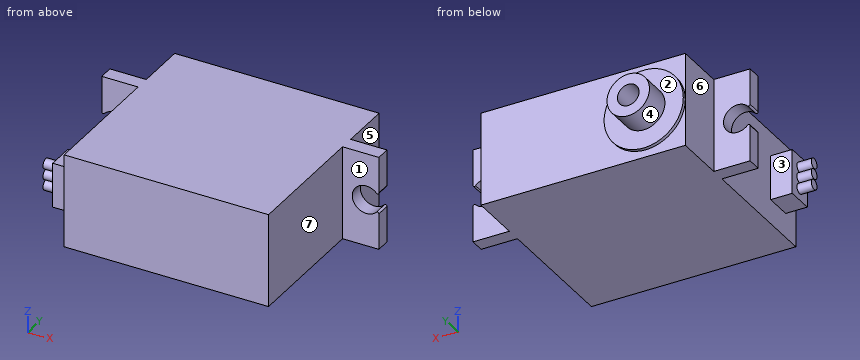
from build123d import *

# Parameters (mm, degrees)
ESQUISSE1_W                       = 28.4
ESQUISSE1_H                       = 27.2
ESQUISSE1_W_2                     = 5.05
ESQUISSE1_H_2                     = 2
BOSS_EXTRU_1_DEPTH                = 6.5
DIAM_TRE_DU_PER_AGE_3_9_3_9_1_D   = 3.9
CONG_1_R                          = 0.2
ESQUISSE6_R                       = 5.5
BOSS_EXTRU_4_DEPTH                = 0.5
ESQUISSE4_R                       = 2.95
BOSS_EXTRU_2_DEPTH                = 3.8
DIAM_TRE_DU_PER_AGE_3_0_3_1_D     = 3
DIAM_TRE_DU_PER_AGE_3_0_3_1_DEPTH = 6
DIAM_TRE_DU_PER_AGE_3_0_3_1_TIP   = 0.901290929
ESQUISSE8_W                       = 6.2
ESQUISSE8_H                       = 3.7
BOSS_EXTRU_5_DEPTH                = 3
ESQUISSE9_R                       = 0.7
BOSS_EXTRU_6_DEPTH                = 2


with BuildPart() as part:
    # Esquisse1 → Boss.-Extru.1 (new, symmetric)
    with BuildSketch(Plane.XY):
        with Locations((0, -4.6)):
            Rectangle(ESQUISSE1_W, ESQUISSE1_H)
        with Locations((-16.725, 1)):
            Rectangle(ESQUISSE1_W_2, ESQUISSE1_H_2)
        with Locations((16.725, 1)):
            Rectangle(ESQUISSE1_W_2, ESQUISSE1_H_2)
    extrude(amount=BOSS_EXTRU_1_DEPTH, both=True)

    # Diamètre du perçage Ø3.9 (3.9)1 (through all)
    with Locations(Plane(origin=(0, 2, 0), x_dir=(1, 0, 0), z_dir=(0, 1, 0))):
        with Locations((-17.5, 0), (17.5, 0)):
            Hole(DIAM_TRE_DU_PER_AGE_3_9_3_9_1_D / 2)

    # Congé1
    cong_1_edges = [part.edges().sort_by_distance(p)[0] for p in [
        (19.25, 1, -0.860232527),
        (19.25, 1, 0.860232527),
        (-19.25, 1, -0.860232527),
        (-19.25, 1, 0.860232527),
    ]]
    fillet(cong_1_edges, radius=CONG_1_R)

    # Esquisse6 → Boss.-Extru.4 (add)
    with BuildSketch(Plane(origin=(0, 9, 0), x_dir=(1, 0, 0), z_dir=(0, 1, 0))):
        with Locations(Location((-8.7, 0, 0), (0, 0, 180))):
            Circle(ESQUISSE6_R)
    extrude(amount=BOSS_EXTRU_4_DEPTH)

    # Esquisse4 → Boss.-Extru.2 (add)
    with BuildSketch(Plane(origin=(0, 9.5, 0), x_dir=(1, 0, 0), z_dir=(0, 1, 0))):
        with Locations((-8.7, 0)):
            Circle(ESQUISSE4_R)
    extrude(amount=BOSS_EXTRU_2_DEPTH)

    # Diamètre du perçage Ø3.0 (3)1
    with Locations(Plane(origin=(0, 13.3, 0), x_dir=(1, 0, 0), z_dir=(0, 1, 0))):
        with Locations((-8.7, 0)):
            Hole(DIAM_TRE_DU_PER_AGE_3_0_3_1_D / 2, depth=DIAM_TRE_DU_PER_AGE_3_0_3_1_DEPTH)
            with Locations((0, 0, -(DIAM_TRE_DU_PER_AGE_3_0_3_1_DEPTH + DIAM_TRE_DU_PER_AGE_3_0_3_1_TIP / 2))):  # 118° drill point
                Cone(0, DIAM_TRE_DU_PER_AGE_3_0_3_1_D / 2, DIAM_TRE_DU_PER_AGE_3_0_3_1_TIP, mode=Mode.SUBTRACT)

    # Esquisse8 → Boss.-Extru.5 (add)
    with BuildSketch(Plane.ZY.offset(14.2)):
        with Locations((0, -13.85)):
            Rectangle(ESQUISSE8_W, ESQUISSE8_H)
    extrude(amount=BOSS_EXTRU_5_DEPTH)

    # Esquisse9 → Boss.-Extru.6 (add)
    with BuildSketch(Plane.ZY.offset(17.2)):
        with Locations((0, -13.85)):
            Circle(ESQUISSE9_R)
        with Locations((-1.5, -13.85)):
            Circle(ESQUISSE9_R)
        with Locations(Location((1.5, -13.85, 0), (0, 0, 180))):
            Circle(ESQUISSE9_R)
    extrude(amount=BOSS_EXTRU_6_DEPTH)


solid = part.part
Geometry: final body of the model. Coordinates: model frame, mm. Face numbers are marked on the shaded views. A direction names the side the tool comes from. Give positions to 0.01 mm unless a question says otherwise; leave off trailing zeros. Order: outer loops, then holes, each group sorted by start corner. A loop starts at its lowest first (then second) coordinate and runs counter-clockwise, first axis right, second up. Notation, with made-up numbers: (-36, 45) -> (-13, 45) arc R12 cw to (-13, 55) -> close; hole circle Ø7 at (52.5, 15). An arc over 180 degrees is marked (long way). Answer as a JSON object with one key per item and string values.
Q1. First-contact query: pin 1 (4.5 mm diameter, centred on x = -17.5, z = 0, fed in from -Y); pin 2 (0.9 mm diameter, centred on x = -15, y = -14, fed in from -Z); pin 3 (4 mm diameter, centred on x = -17, z = 1.5, fed in from +Y). Flat tips, straight axial feed; report the tip coordinate or a pass-through.
Entries:
{"pin 1": "stops at y = -15.7", "pin 2": "stops at z = -3.1", "pin 3": "stops at y = 2"}
Q2. Section D-D (x = -15). Output: boundary loops of the cut face in (y, z), plus the area to 3 significant figures.
Entries:
{"outline": "(-15.7, -3.1) -> (-12, -3.1) -> (-12, 3.1) -> (-15.7, 3.1) -> close; (0, -6.5) -> (2, -6.5) -> (2, 6.5) -> (0, 6.5) -> close", "area": "48.9 mm^2"}
Q3. Material intervals for probe 1 along X at (y, z) = (-12.5, -2.5); probe 2 along X at (y, z) = (-7, -5); probe 3 along Y at (x, z) = (-15, 1.5), sorted ascending.
Entries:
{"probe 1": "x = -17.2 to 14.2", "probe 2": "x = -14.2 to 14.2", "probe 3": "y = -15.7 to -12, 0 to 2"}
Q4. Section B-B (y = -13.85). Output: boundary loops of the cut face in (x, z).
Entries:
{"outline": "(-19.2, -2.2) -> (-17.2, -2.2) -> (-17.2, -3.1) -> (-14.2, -3.1) -> (-14.2, -6.5) -> (14.2, -6.5) -> (14.2, 6.5) -> (-14.2, 6.5) -> (-14.2, 3.1) -> (-17.2, 3.1) -> (-17.2, 2.2) -> (-19.2, 2.2) -> (-19.2, 0.8) -> (-17.2, 0.8) -> (-17.2, 0.7) -> (-19.2, 0.7) -> (-19.2, -0.7) -> (-17.2, -0.7) -> (-17.2, -0.8) -> (-19.2, -0.8) -> close"}
Q5. Section C-C (z = 4.5). Output: boundary loops of the cut face in (x, y).
Entries:
{"outline": "(-19.25, 0) -> (-14.2, 0) -> (-14.2, -18.2) -> (14.2, -18.2) -> (14.2, 0) -> (19.25, 0) -> (19.25, 2) -> (14.2, 2) -> (14.2, 9) -> (-5.54, 9) -> (-5.54, 9.5) -> (-11.86, 9.5) -> (-11.86, 9) -> (-14.2, 9) -> (-14.2, 2) -> (-19.25, 2) -> close"}
Q6. Access query for the marked faces 4, 5, 6 and 7. Directions: +Z, -Z, +X, -X, +Y, -Y. A direction counts if a zero-diameter tool reaches every point of the face in a straight line with its end or side. Return the directions, or none.
Entries:
{"face 4": "+Y", "face 5": "+Z, -Z, +X, +Y", "face 6": "+Z, -Z, -X, +Y", "face 7": "+Z, -Z, +X, -Y"}
Q7. Section A-A (x = 17.5). Output: boundary loops of the cut face in (y, z), plus the area to 3 significant figures.
Entries:
{"outline": "(0, -6.5) -> (2, -6.5) -> (2, -1.95) -> (0, -1.95) -> close; (0, 1.95) -> (2, 1.95) -> (2, 6.5) -> (0, 6.5) -> close", "area": "18.2 mm^2"}
Q8. Draft query along Y for the marked faces 1, 2 and 3. Return one class per face: released by +Y, released by -Y, zero draft, split by the parting line, or undercut.
Entries:
{"face 1": "released by -Y", "face 2": "released by +Y", "face 3": "undercut"}
